Autodesk Inventor part; units mm, degrees
ref_plane "YZ Plane" through (0, 0, 0) normal (1, 0, 0) x (0, 1, 0)
ref_plane "XZ Plane" through (0, 0, 0) normal (0, 1, 0) x (-1, 0, 0)
ref_plane "XY Plane" through (0, 0, 0) normal (0, 0, 1) x (1, 0, 0)
ref_plane "Arbeitsebene2" through (0, 0, 0) normal (0, 0, -1) x (0, 1, 0)
sketch "Skizze6" plane through (0, 0, 0) normal (0, 0, -1) x (0, 1, 0)
  circle A0 centre (0, 25) radius 1.95
  circle A1 centre (-25, 0) radius 1.95
  circle A2 centre (-25, -25) radius 1.95
  circle A3 centre (25, 25) radius 1.95
  circle A4 centre (25, -25) radius 1.95
  circle A5 centre (-25, 25) radius 1.95
  circle A6 centre (25, 0) radius 1.95
  circle A7 centre (0, -25) radius 1.95
  line L0 (-28, 30) -> (-30, 28)
  line L1 (-30, 28) -> (-30, -28)
  line L2 (-30, -28) -> (-28, -30)
  line L3 (-28, -30) -> (28, -30)
  line L4 (28, -30) -> (30, -28)
  line L5 (30, -28) -> (30, 28)
  line L6 (30, 28) -> (28, 30)
  line L7 (28, 30) -> (-28, 30)
  line L8 (-40.5166, -48.4344) -> (-70.5166, -48.4344) construction
  line L9 (-70.5166, -48.4344) -> (-70.5166, -78.4344) construction
  line L10 (-70.5166, -78.4344) -> (-40.5166, -78.4344) construction
  line L11 (-40.5166, -78.4344) -> (-40.5166, -48.4344) construction
  line L12 (-40.5166, -48.4344) -> (-70.5166, -78.4344) construction
  line L13 (-70.5166, -48.4344) -> (-40.5166, -78.4344) construction
  line L14 (-75, -48) -> (-45, -48)
  line L15 (-45, -48) -> (-45, -78)
  line L16 (-45, -78) -> (-75, -78)
  line L17 (-75, -78) -> (-75, -48)
  line L18 (-75, -48) -> (-45, -78) construction
  line L19 (-45, -48) -> (-75, -78) construction
  line L20 (-45, -48) -> (-30, -48)
  line L21 (-30, -48) -> (-30, -28)
  line L22 (-45, -78) -> (0, -78)
  line L23 (0, -78) -> (0, -30)
  circle A8 centre (-55.5095, -63.317) radius 8.4793
  line L24 (-28, 30) -> (-75, 30)
  line L25 (-75, 30) -> (-75, -48)
  line L26 (-28, -30) -> (-45, -30)
  line L27 (-45, -30) -> (-45, -48)
  line L28 (-45, -78) -> (-37, -78)
  line L29 (-37, -78) -> (-37, -48)
  line L30 (-37, -48) -> (-45, -48)
  line L31 (-45, -48) -> (-45, -78)
  line L32 (-45, -30) -> (-37, -30)
  line L33 (-37, -30) -> (-37, -48)
  line L34 (-37, -48) -> (-45, -48)
  line L35 (-45, -48) -> (-45, -30)
  point P0 (0, 0)
  point P1 (-55.5166, -63.4344)
  point P2 (-60, -63)
  dimension "d10" = 30
  dimension "d11" = 30
  dimension "d12" = 30
  dimension "d13" = 30
  dimension "d14" = 45
  dimension "d15" = 18
  dimension "d28" = 8
extrude "Extrusion1" add sketch "Skizze6" along normal blind 12 contours L7 L6 L5 L4 L3 L2 L1 L0 | L0 L1 L21 L26 L27 L14 L25 L24 | L2 L26 L21 | L14 L15 L16 L17 | L20 L29 L22 L15 | L27 L26 L33 L20 | A8
chamfer "Fase1" distance 2 angle 45 4 edges at (-78, -75, -6) (30, -75, -6) (-30, -37, -6) (-78, -37, -6)
sketch "Skizze7" plane through (0, 0, -12) normal (0, 0, -1) x (-1, 0, 0)
  line L0 (30, -35) -> (30, 28)
  line L1 (30, 28) -> (28, 30)
  line L2 (28, 30) -> (-28, 30)
  line L3 (-28, 30) -> (-30, 28)
  line L4 (-30, 28) -> (-30, -73)
  circle A0 centre (25, 0) radius 1.95
  circle A1 centre (0, 25) radius 1.95
  circle A2 centre (-25, -25) radius 1.95
  circle A3 centre (25, 25) radius 1.95
  circle A4 centre (-25, 25) radius 1.95
  circle A5 centre (25, -25) radius 1.95
  circle A6 centre (0, -25) radius 1.95
  circle A7 centre (-25, 0) radius 1.95
  line L5 (78, -73) -> (76, -75)
  line L6 (-28, -75) -> (76, -75)
  line L7 (-28, -75) -> (-30, -73)
  line L8 (78, -73) -> (78, -39)
  line L9 (76, -37) -> (32, -37)
  line L10 (76, -37) -> (78, -39)
  line L11 (30, -35) -> (32, -37)
  point P0 (0, 0)
hole "Bohrung2" at (-25, 25, -12) at (-25, 0, -12) at (-25, -25, -12) at (25, -25, -12) at (25, 0, -12) at (25, 25, -12) at (0, 25, -12) at (0, -25, -12) direction (0, 0, 1) diameter 5 end through all counterbore diameter 8 counterbore depth 5
sketch "Skizze8" plane through (0, 0, 0) normal (0, 0, 1) x (1, 0, 0)
  circle A0 centre (-63.4834, -64.233) radius 2.95
  circle A1 centre (-75.6078, -43.5) radius 2.95
  circle A2 centre (-51.3591, -43.5) radius 2.95
  point P0 (0, 0)
hole "Bohrung3" at (-51.3591, -43.5, 0) at (-63.4834, -64.233, 0) at (-75.6078, -43.5, 0) direction (0, 0, -1) diameter 2.8 end through all counterbore diameter 6.5 counterbore depth 3
equation "\"BendRadius\" = Thickness"
equation "\"BendReliefWidth\" = Thickness"
equation "\"BendReliefDepth\" = 0.5 * Thickness"
equation "\"CornerReliefSize\" = 4 * Thickness"
equation "\"MinimumRemnant\" = 2 * Thickness"
equation "\"TransitionRadius\" = BendRadius"
equation "\"JacobiRadiusSize\" = Thickness"
equation "\"GapSize\" = Thickness"
properties part number "cellSTORM_Base_v0_R1"
Geometry check sheet. Reference: the model listing, model coordinates, mm. A direction names the side the tool comes from. Round coordinates to 2 decimals unless told otherwise and drop trailing zeros. Loops run counter-clockwise (first coordinate to the right, second up) from the corner with the lowest first, then second, coordinate; pieces in that order, holes last. Notation, with made-up numbers: (69, 74.5) - (126, 74.5) arc R25 cw to (126, 87.5) - close; hole circle Ø10 at (80.5, 1.25). An arc over 180 degrees is marked (long way). Use a Markdown table: item, result.
Q1. Cross-section at B-B on x = 25. Record the cut outline in (y, z), plus the area to 4 significant figures.
Solutions:
| item | result |
|---|---|
| outline | (-75, -12) - (-29, -12) - (-29, -7) - (-27.5, -7) - (-27.5, 0) - (-75, 0) - close; (-22.5, -7) - (-21, -7) - (-21, -12) - (-4, -12) - (-4, -7) - (-2.5, -7) - (-2.5, 0) - (-22.5, 0) - close; (2.5, -7) - (4, -7) - (4, -12) - (21, -12) - (21, -7) - (22.5, -7) - (22.5, 0) - (2.5, 0) - close; (27.5, -7) - (29, -7) - (29, -12) - (30, -12) - (30, 0) - (27.5, 0) - close |
| area | 1,035 mm2 |
Q2. Draft check along X on faces 1 (the cylindrical face through (-0.1, -27.5, -3.5)), 2 (the flat face through (-30, -4, -6)), 3 (the flat face through (-54, -37, -6)). Enter one of: released by +X, released by -X, zero draft, split by the parting line, or undercut.
Solutions:
| item | result |
|---|---|
| face 1 | undercut |
| face 2 | released by -X |
| face 3 | zero draft |
Q3. Cross-section at C-C on x = 0. Record the cut outline in (y, z).
Solutions:
| item | result |
|---|---|
| outline | (-75, -12) - (-29, -12) - (-29, -7) - (-27.5, -7) - (-27.5, 0) - (-75, 0) - close; (-22.5, -7) - (-21, -7) - (-21, -12) - (21, -12) - (21, -7) - (22.5, -7) - (22.5, 0) - (-22.5, 0) - close; (27.5, -7) - (29, -7) - (29, -12) - (30, -12) - (30, 0) - (27.5, 0) - close |
Q4. Material ranges on line 1 (Y direction, x = 0, z = -4); line 2 (X direction, y = 0, z = -8.3); line 3 (Y direction, x = 0, z = -9.45), recorded low to high.
Solutions:
| item | result |
|---|---|
| line 1 | y = -75 to -27.5, -22.5 to 22.5, 27.5 to 30 |
| line 2 | x = -30 to -29, -21 to 21, 29 to 30 |
| line 3 | y = -75 to -29, -21 to 21, 29 to 30 |
Q5. Go/stop test with flat-tipped pins: P1, Ø2.5, axis at x = -23, y = 26.5, coming from the -Z side; P2, Ø2, axis at x = -62.5, y = -65, coming from the +Z side. Record where each tip stops, or that it passes through.
Solutions:
| item | result |
|---|---|
| P1 | stops at z = -7 |
| P2 | stops at z = -3 |
Q6. Access from +Z, -Z, +X, -X, +Y, -Y to the whole of each face (thin tool, end or side, straight path). Record for faces 4 (the cylindrical face through (-49.99, -43.2, -7.56)), 5 (the flat face through (-49.96, -44.18, -3)), 6 (the flat face through (23, -23, -7)).
Solutions:
| item | result |
|---|---|
| face 4 | +Z, -Z |
| face 5 | +Z |
| face 6 | -Z |
Q7. Cross-section at D-D on y = 25. Record the cut outline in (x, z), plus the area to 3 significant figures.
Solutions:
| item | result |
|---|---|
| outline | (-30, -12) - (-29, -12) - (-29, -7) - (-27.5, -7) - (-27.5, 0) - (-30, 0) - close; (-22.5, -7) - (-21, -7) - (-21, -12) - (-4, -12) - (-4, -7) - (-2.5, -7) - (-2.5, 0) - (-22.5, 0) - close; (2.5, -7) - (4, -7) - (4, -12) - (21, -12) - (21, -7) - (22.5, -7) - (22.5, 0) - (2.5, 0) - close; (27.5, -7) - (29, -7) - (29, -12) - (30, -12) - (30, 0) - (27.5, 0) - close |
| area | 495 mm2 |
Q8. Cross-section at A-A on y = 0. Record the cut outline in (x, z).
Solutions:
| item | result |
|---|---|
| outline | (-30, -12) - (-29, -12) - (-29, -7) - (-27.5, -7) - (-27.5, 0) - (-30, 0) - close; (-22.5, -7) - (-21, -7) - (-21, -12) - (21, -12) - (21, -7) - (22.5, -7) - (22.5, 0) - (-22.5, 0) - close; (27.5, -7) - (29, -7) - (29, -12) - (30, -12) - (30, 0) - (27.5, 0) - close |
